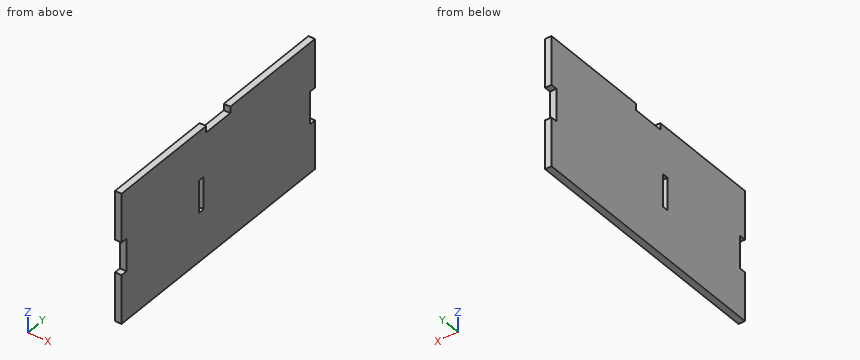
```python
from build123d import *

# Parameters (mm, degrees)
F0_W     = 5
F0_H     = 25
F1_DEPTH = 5


# Not quite as in the source:
# - a feature names something its author has since deleted; it is built from what else it names


with BuildPart() as f1:
    # F0 (on Right) → F1 (new body)
    with BuildSketch(Plane.YZ):
        Polygon((138.9010111106, 39.8091464203), (138.9010111106, 77.3091464203), (51.4010111106, 77.3091464203), (51.4010111106, 72.3091464203), (26.4010111106, 72.3091464203), (26.4010111106, 77.3091464203), (-61.0989888894, 77.3091464203), (-61.0989888894, 39.8091464203), (-56.0989888894, 39.8091464203), (-56.0989888894, 14.8091464203), (-61.0989888894, 14.8091464203), (-61.0989888894, -22.6908535797), (138.9010111106, -22.6908535797), (138.9010111106, 14.8091464203), (133.9010111106, 14.8091464203), (133.9010111106, 39.8091464203), align=None)
        with Locations((21.4010111106, 27.3091464203)):
            Rectangle(F0_W, F0_H, mode=Mode.SUBTRACT)
    extrude(amount=F1_DEPTH)


solid = f1.part
```
Here's how the part is built. I have some questions about the finished solid (model axes, mm). Coordinates: 2 decimals unless noted, no trailing zeros. Order: outer loops, then holes, each group sorted by start corner. A loop starts at its lowest first (then second) coordinate and runs counter-clockwise, first axis right, second up.
1) Imagine slicing it at B-B on x = 3.55. List the corners of the cut face in (y, z) for me.
2) Will these pins go through, and if not, where does the flat tip stop? pin 1 (1.5 mm diameter, centred on x = 1.5, y = 45, fed in from +Z); pin 2 (2.5 mm diameter, centred on x = 1.5, z = 31, fed in from +Y); pin 3 (1.5 mm diameter, centred on x = 1.5, z = 24, fed in from -Y).
3) I need wall thicknesses on line 1 (Y direction, x = 0.3, z = 24); line 2 (Z direction, x = 2.7, y = 21); line 3 (Z direction, x = 1.5, y = 33.5). Which ranges of each line are inside material? Lowest first, please.
4) Imagine slicing it at A-A on z = 18. List the corners of the cut face in (x, y) for me, and give its area (3 significant figures).
Response values:
1. outline: (-61.1, -22.69) - (138.9, -22.69) - (138.9, 14.81) - (133.9, 14.81) - (133.9, 39.81) - (138.9, 39.81) - (138.9, 77.31) - (51.4, 77.31) - (51.4, 72.31) - (26.4, 72.31) - (26.4, 77.31) - (-61.1, 77.31) - (-61.1, 39.81) - (-56.1, 39.81) - (-56.1, 14.81) - (-61.1, 14.81) - close; hole (18.9, 14.81) - (23.9, 14.81) - (23.9, 39.81) - (18.9, 39.81) - close
2. pin 1: stops at z = 72.31
2. pin 2: stops at y = 133.9
2. pin 3: stops at y = -56.1
3. line 1: y = -56.1 to 18.9, 23.9 to 133.9
3. line 2: z = -22.69 to 14.81, 39.81 to 77.31
3. line 3: z = -22.69 to 72.31
4. outline: (0, -56.1) - (5, -56.1) - (5, 18.9) - (0, 18.9) - close; (0, 23.9) - (5, 23.9) - (5, 133.9) - (0, 133.9) - close
4. area: 925 mm2
